Geometry: final body of the model. Coordinates: model frame, mm. Give positions to 0.01 mm unless a question says otherwise; leave off trailing zeros. Loops run counter-clockwise (first coordinate to the right, second up) from the corner with the lowest first, then second, coordinate; pieces in that order, holes last.
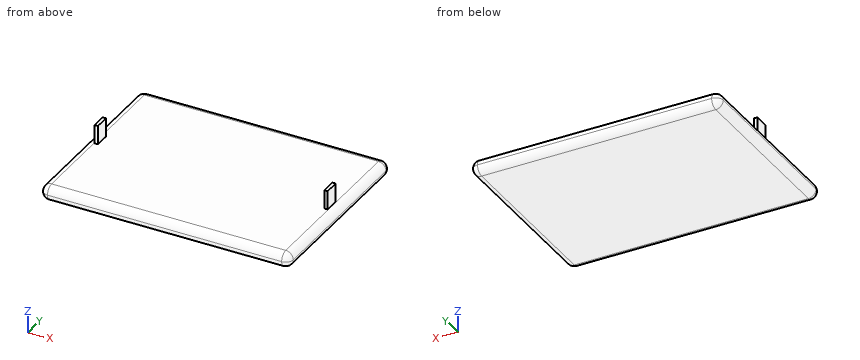
from build123d import *

# Parameters (mm, degrees)
F0_W     = 167.9448
F0_H     = 10.16
F1_DEPTH = 62.484
F2_W     = 2.2802874446
F2_H     = 9.9761183374
F3_DEPTH = 12.7
F4_R     = 5.07999


# Not quite as in the source:
# - a fillet or chamfer is up to 0.001 mm smaller than in the source, because OpenCascade refuses the exact size


with BuildPart() as f1:
    # F0 (on Front) → F1 (new body, symmetric)
    with BuildSketch(Plane.XZ):
        Rectangle(F0_W, F0_H)
    extrude(amount=F1_DEPTH, both=True)

    # F2 (on face) → F3 (join)
    with BuildSketch(Plane.XY.offset(5.08)):
        with Locations((-77.4024613202, 0.1807718072)):
            Rectangle(F2_W, F2_H)
        with Locations((77.4024613202, 0.1807718072)):
            Rectangle(F2_W, F2_H)
    extrude(amount=F3_DEPTH)

    # F4 (radius 5.08 in the source; OpenCascade refuses exactly that, so slightly less here)
    f4_edges = [f1.edges().sort_by_distance(p)[0] for p in [
        (0, -62.484, 5.08),
        (-83.9724, -62.484, 0),
        (0, -62.484, -5.08),
        (83.9724, -62.484, 0),
        (83.9724, 0, 5.08),
        (-83.9724, 0, 5.08),
        (0, 62.484, 5.08),
        (-83.9724, 0, -5.08),
        (0, 62.484, -5.08),
        (83.9724, 0, -5.08),
        (83.9724, 62.484, 0),
        (-83.9724, 62.484, 0),
    ]]
    fillet(f4_edges, radius=F4_R)


solid = f1.part
Item 1: Section query D-D on z = 2.75. Return loops of the section in (x, y), plus the area to 3 significant figures.
Values follow:
outline: (-83.16, -57.4) arc R4.27 ccw to (-78.89, -61.68) - (78.89, -61.68) arc R4.27 ccw to (83.16, -57.4) - (83.16, 57.4) arc R4.27 ccw to (78.89, 61.68) - (-78.89, 61.68) arc R4.27 ccw to (-83.16, 57.4) - close
area: 20,500 mm2
Item 2: Ray query, probe 1 along X at (y, z) = (-2, 9.25); probe 2 along X at (y, z) = (-16, -0.5); probe 3 along Z at (x, y) = (-57.5, -30.5). Return the intervals inside material, ascending.
Values follow:
probe 1: x = -78.54 to -76.26, 76.26 to 78.54
probe 2: x = -83.95 to 83.95
probe 3: z = -5.08 to 5.08
Item 3: Pin query (flat end, axial travel): pin 1 (0.7 mm diameter, centred on x = 77.5, z = 11, fed in from +Y); pin 2 (1.1 mm diameter, centred on x = -77.5, z = 9.5, fed in from -Y); pin 3 (1.5 mm diameter, centred on x = 47, y = -22, fed in from +Z). Return the tip coordinate at first contact, or that it passes through.
Values follow:
pin 1: stops at y = 5.17
pin 2: stops at y = -4.81
pin 3: stops at z = 5.08
Item 4: Section query A-A on z = 10.5. Return loops of the section in (x, y), plus the area to 3 significant figures.
Values follow:
outline: (-78.54, -4.81) - (-76.26, -4.81) - (-76.26, 5.17) - (-78.54, 5.17) - close; (76.26, -4.81) - (78.54, -4.81) - (78.54, 5.17) - (76.26, 5.17) - close
area: 45.5 mm2
